The listing builds one solid part. Answer for the finished solid, in the listing's coordinates (mm). A direction names the side the tool comes from. Give positions to 0.01 mm unless a question says otherwise; leave off trailing zeros. Order: outer loops, then holes, each group sorted by start corner. A loop starts at its lowest first (then second) coordinate and runs counter-clockwise, first axis right, second up. Notation, with made-up numbers: (-13.75, 29.5) - (-6.75, 29.5) arc R17 ccw to (-6.75, 62.5) - close; hole circle Ø10 at (41, -20.5). An arc over 180 degrees is marked (long way). Answer in a Markdown table with one row per item. Add a question column.
```python
from build123d import *

# Parameters (mm, degrees)
BOSS_EXTRUDE2_DEPTH = 3.175


with BuildPart() as part:
    # Sketch1 → Boss-Extrude2 (new body)
    with BuildSketch(Plane(origin=(0, 0, 0), x_dir=(1, 0, 0), z_dir=(0, 1, 0))):
        Polygon((-19.05, -34.925), (-19.05, -31.75), (-26.67, -31.75), (-26.67, -34.925), (-34.29, -34.925), (-34.29, -31.75), (-38.1, -31.75), (-38.1, 34.925), (-6.35, 34.925), (-6.35, 31.75), (6.35, 31.75), (6.35, 34.925), (38.1, 34.925), (38.1, -31.75), (34.29, -31.75), (34.29, -34.925), (26.67, -34.925), (26.67, -31.75), (19.05, -31.75), (19.05, -34.925), (11.43, -34.925), (11.43, -31.75), (3.81, -31.75), (3.81, -34.925), (-3.81, -34.925), (-3.81, -31.75), (-11.43, -31.75), (-11.43, -34.925), align=None)
        Polygon((-30.998556448, -5.5626), (-30.082012895, -3.9751), (-30.998556448, -2.3876), (-32.831643552, -2.3876), (-33.748187105, -3.9751), (-32.831643552, -5.5626), align=None, mode=Mode.SUBTRACT)
        Polygon((-30.082012895, 26.5049), (-30.998556448, 28.0924), (-32.831643552, 28.0924), (-33.748187105, 26.5049), (-32.831643552, 24.9174), (-30.998556448, 24.9174), align=None, mode=Mode.SUBTRACT)
        Polygon((32.831643552, 24.9174), (33.748187105, 26.5049), (32.831643552, 28.0924), (30.998556448, 28.0924), (30.082012895, 26.5049), (30.998556448, 24.9174), align=None, mode=Mode.SUBTRACT)
        Polygon((-6.233556448, -27.7876), (-5.317012895, -26.2001), (-6.233556448, -24.6126), (-8.066643552, -24.6126), (-8.983187105, -26.2001), (-8.066643552, -27.7876), align=None, mode=Mode.SUBTRACT)
        Polygon((33.748187105, -26.5303), (32.831643552, -24.9428), (30.998556448, -24.9428), (30.082012895, -26.5303), (30.998556448, -28.1178), (32.831643552, -28.1178), align=None, mode=Mode.SUBTRACT)
    extrude(amount=BOSS_EXTRUDE2_DEPTH)


solid = part.part
```
(1) Straight lines are drawn through the part: line 1 (X direction, y = 1.95, z = 26); line 2 (Z direction, x = -7.5, y = 1.45) (3 decimals); line 3 (X direction, y = 1.3, z = 4). For each, find the intervals that lie inside material, in ascending order.
(2) Each of these flat-tipped pins is pushed along its axis until it touches: P1, Ø1.6, axis at y = 1.5, z = 33, coming from the -X side; P2, Ø1, axis at x = 37, y = 1.5, coming from the +Z side. Where does it stop, or does it pass through?
(3) Find section B-B, the plane y = 0.5. Give the number of separate pieces and of enclosed holes in the cut face, plus the area to 3 significant figures.
(4) The mould has two halves that part along Z. Classify faces 5 (the face through (23, 2, 31.75)), 6 (the face through (-30.547, 1.565, 4.78)), 7 (the face through (1, 0, 0)): +Z half, -Z half, draft (parallel to the pull), parting line (faces both ways), or undercut.
(5) For faces 1 (the face through (11.43, 2, 33)), 2 (the face through (0, 2, 34.925)), 3 (the face through (-30.547, 1.565, -25.7)), 4 (the face through (36, 2, 31.75)), determine the directions among +Z, -Z, +X, -X, +Y, -Y from which every point of the face is accessible in a straight line to the end or side of a thin tool.
(6) Find section A-A, the plane x = 24. Write down the section's boundary in (y, z) (3 decimals).
Answer key:
| question | item | result |
|---|---|---|
| 1 | line 1 | -38.1 to -8.87, -5.43 to 30.39, 33.44 to 38.1 |
| 1 | line 2 | -34.925 to 24.613, 27.788 to 31.75 |
| 1 | line 3 | -38.1 to -33.73, -30.1 to 38.1 |
| 2 | P1 | x = -34.29 |
| 2 | P2 | z = 31.75 |
| 3 | separate pieces | 1 |
| 3 | enclosed holes | 5 |
| 3 | area | 5,120 mm² |
| 4 | face 5 | +Z half |
| 4 | face 6 | undercut |
| 4 | face 7 | draft |
| 5 | face 1 | +Z, +Y, -Y |
| 5 | face 2 | +Z, +X, -X, +Y, -Y |
| 5 | face 3 | +Y, -Y |
| 5 | face 4 | +Z, +X, +Y, -Y |
| 6 | outline | (0, -34.925) - (3.175, -34.925) - (3.175, 31.75) - (0, 31.75) - close |
